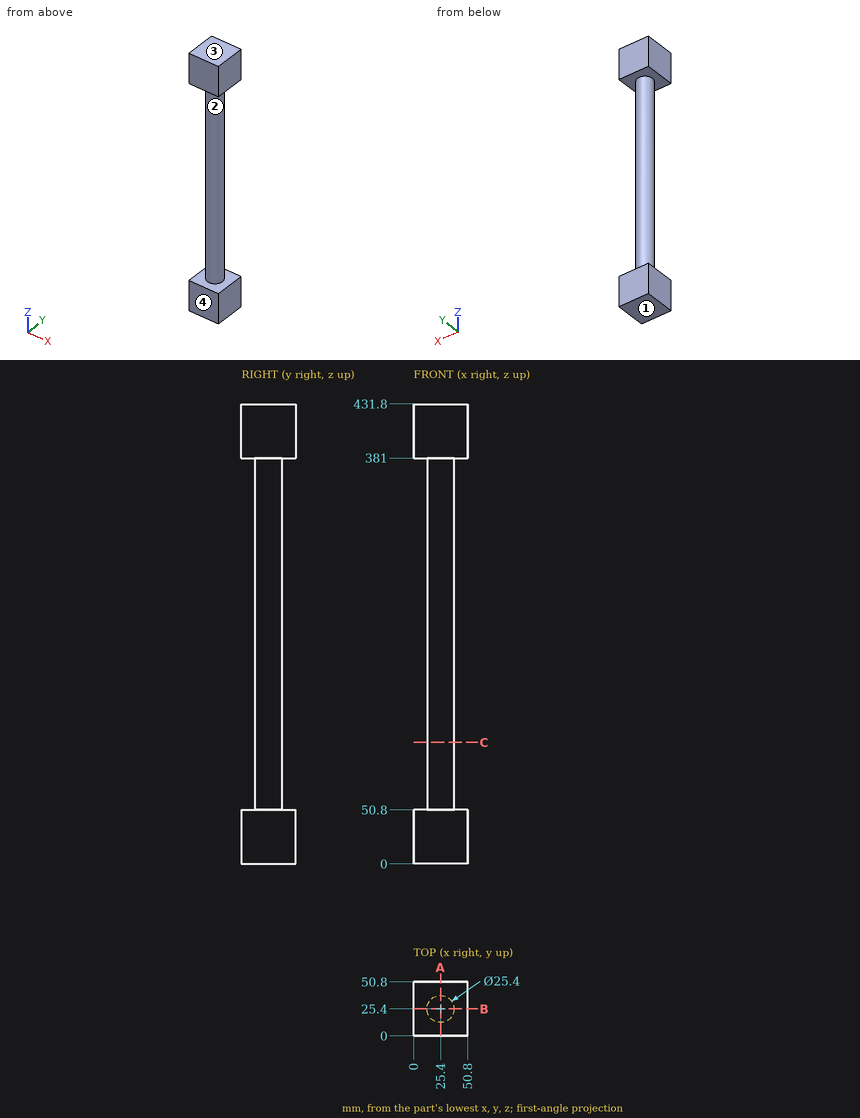
Check sheet for the drawn part. Datum: minimum x, y, z corner. Units: mm. Give positions to 0.01 mm unless a question says otherwise; leave off trailing zeros. Order: outer loops, then holes, each group sorted by start corner. A loop starts at its lowest first (then second) coordinate and runs counter-clockwise, first axis right, second up.
1. Draft check along Z on the marked faces 1, 2, 3 and 4. Enter one of: pulls with the +Z half, pulls with the -Z half, needs draft (parallel to the pull), parting line crosses it, or undercut.
Completed:
face 1: pulls with the -Z half
face 2: undercut
face 3: pulls with the +Z half
face 4: needs draft
2. Sectioned sample at C-C (z = 114). Record the boundary of the cut face in (x, y), then the cut area to 3 significant figures.
Completed:
outline: circle Ø25.4 at (25.4, 25.4)
area: 507 mm2
3. Scan lines: line 1 (Z direction, x = 45, y = 45); line 2 (Y direction, x = 20, z = 343); line 3 (Y direction, x = 29, z = 201.5). Record each from-to range of solid material in increasing order.
Completed:
line 1: z = 0 to 50.8, 381 to 431.8
line 2: y = 13.91 to 36.89
line 3: y = 13.22 to 37.58
4. Sectioned sample at A-A (x = 25.4). Record the boundary of the cut face in (y, z), then the cut area to 3 significant figures.
Completed:
outline: (0, 0) - (50.8, 0) - (50.8, 50.8) - (38.1, 50.8) - (38.1, 381) - (50.8, 381) - (50.8, 431.8) - (0, 431.8) - (0, 381) - (12.7, 381) - (12.7, 50.8) - (0, 50.8) - close
area: 13,500 mm2
5. Depth check by flat-ended pin: pin 1 (3 mm diameter, centred on y = 10, z = 358.5, fed in from +X); pin 2 (6 mm diameter, centred on y = 17, z = 215, fed in from +X); pin 3 (4 mm diameter, centred on y = 31.5, z = 140, fed in from -X); pin 4 (3 mm diameter, centred on y = 36, z = 85, fed in from +X). Enter the tip coordinate at first touch or a pass-through.
Completed:
pin 1: passes through
pin 2: stops at x = 36.89
pin 3: stops at x = 13.38
pin 4: stops at x = 34.26
